Build history of the part. All positions in model axes, mm. A direction names the side the tool comes from. Round coordinates to 2 decimals unless told otherwise and drop trailing zeros. Write each loop counter-clockwise with the first axis right and the second up, starting at its lowest first coordinate (ties: lowest second). Pieces come first, ordered by that corner, then holes. Notation, with made-up numbers: (56, 35) - (103, 35) arc R15 ccw to (103, 55) - close; hole circle Ø3 at (86.25, 88). An arc over 180 degrees is marked (long way). One line per question, with ' | ' between items.
from build123d import *

# Parameters (mm, degrees)
BOSS_EXTRUDE1_DEPTH = 5
BOSS_EXTRUDE2_DEPTH = 1
SKETCH3_R           = 0.75
BOSS_EXTRUDE3_DEPTH = 2
CUT_EXTRUDE1_START  = -3
SKETCH4_R           = 0.75
CUT_EXTRUDE1_DEPTH  = 3


with BuildPart() as part:
    # Sketch1 → Boss-Extrude1 (new body)
    with BuildSketch(Plane.XY):
        Polygon((0, 57.735026919), (-50, 28.867513459), (-50, -28.867513459), (0, -57.735026919), (50, -28.867513459), (50, 28.867513459), align=None)
        Polygon((0, 54.270925304), (-47, 27.135462652), (-47, -27.135462652), (0, -54.270925304), (47, -27.135462652), (47, 27.135462652), align=None, mode=Mode.SUBTRACT)
    extrude(amount=BOSS_EXTRUDE1_DEPTH)

    # Sketch2 → Boss-Extrude2 (add)
    with BuildSketch(Plane(origin=(0, 0, 0), x_dir=(-1, 0, 0), z_dir=(0, 0, -1))):
        Polygon((-47, -27.135462652), (-47, 27.135462652), (0, 54.270925304), (47, 27.135462652), (47, -27.135462652), (0, -54.270925304), align=None)
    extrude(amount=-BOSS_EXTRUDE2_DEPTH)

    # Sketch3 → Boss-Extrude3 (add)
    # profile 1 of 6: a face of its own
    with BuildSketch(Plane.XY.offset(5)):
        with BuildLine():
            Line((1.5, 56.002976111), (1.5, 56.869001515))
            Line((1.5, 56.869001515), (0, 57.735026919))
            Line((0, 57.735026919), (-1.5, 56.869001515))
            Line((-1.5, 56.869001515), (-1.5, 56.002976111))
            ThreePointArc((-1.5, 56.002976111), (0, 54.502976111), (1.5, 56.002976111))
        make_face()
        with Locations((0, 56.002976111)):
            Circle(SKETCH3_R, mode=Mode.SUBTRACT)
    # profile 2 of 6: a face of its own
    with BuildSketch(Plane.XY.offset(5)):
        with BuildLine():
            Line((50, 27.135462652), (50, 28.867513459))
            Line((50, 28.867513459), (48.5, 29.733538863))
            Line((48.5, 29.733538863), (47.75, 29.300526161))
            ThreePointArc((47.75, 29.300526161), (47.200961894, 27.251488056), (49.25, 26.70244995))
            Line((49.25, 26.70244995), (50, 27.135462652))
        make_face()
        with Locations((48.5, 28.001488056)):
            Circle(SKETCH3_R, mode=Mode.SUBTRACT)
    # profile 3 of 6: a face of its own
    with BuildSketch(Plane.XY.offset(5)):
        with BuildLine():
            Line((50, -28.867513459), (50, -27.135462652))
            Line((50, -27.135462652), (49.25, -26.70244995))
            ThreePointArc((49.25, -26.70244995), (47.200961894, -27.251488056), (47.75, -29.300526161))
            Line((47.75, -29.300526161), (48.5, -29.733538863))
            Line((48.5, -29.733538863), (50, -28.867513459))
        make_face()
        with Locations((48.5, -28.001488056)):
            Circle(SKETCH3_R, mode=Mode.SUBTRACT)
    # profile 4 of 6: a face of its own
    with BuildSketch(Plane.XY.offset(5)):
        with BuildLine():
            Line((0, -57.735026919), (1.5, -56.869001515))
            Line((1.5, -56.869001515), (1.5, -56.002976111))
            ThreePointArc((1.5, -56.002976111), (0, -54.502976111), (-1.5, -56.002976111))
            Line((-1.5, -56.002976111), (-1.5, -56.869001515))
            Line((-1.5, -56.869001515), (0, -57.735026919))
        make_face()
        with Locations((0, -56.002976111)):
            Circle(SKETCH3_R, mode=Mode.SUBTRACT)
    # profile 5 of 6: a face of its own
    with BuildSketch(Plane.XY.offset(5)):
        with BuildLine():
            Line((-50, -28.867513459), (-48.5, -29.733538863))
            Line((-48.5, -29.733538863), (-47.75, -29.300526161))
            ThreePointArc((-47.75, -29.300526161), (-47.200961894, -27.251488056), (-49.25, -26.70244995))
            Line((-49.25, -26.70244995), (-50, -27.135462652))
            Line((-50, -27.135462652), (-50, -28.867513459))
        make_face()
        with Locations((-48.5, -28.001488056)):
            Circle(SKETCH3_R, mode=Mode.SUBTRACT)
    # profile 6 of 6: a face of its own
    with BuildSketch(Plane.XY.offset(5)):
        with BuildLine():
            Line((-47.75, 29.300526161), (-48.5, 29.733538863))
            Line((-48.5, 29.733538863), (-50, 28.867513459))
            Line((-50, 28.867513459), (-50, 27.135462652))
            Line((-50, 27.135462652), (-49.25, 26.70244995))
            ThreePointArc((-49.25, 26.70244995), (-47.200961894, 27.251488056), (-47.75, 29.300526161))
        make_face()
        with Locations((-48.5, 28.001488056)):
            Circle(SKETCH3_R, mode=Mode.SUBTRACT)
    extrude(amount=BOSS_EXTRUDE3_DEPTH)

    # Sketch4 → Cut-Extrude1 (cut)
    with BuildSketch(Plane.XY.offset(5).offset(CUT_EXTRUDE1_START)):
        with Locations((0, 56.002976111)):
            Circle(SKETCH4_R)
        with Locations((-48.5, 28.001488056)):
            Circle(SKETCH4_R)
        with Locations((-48.5, -28.001488056)):
            Circle(SKETCH4_R)
        with Locations((0, -56.002976111)):
            Circle(SKETCH4_R)
        with Locations((48.5, -28.001488056)):
            Circle(SKETCH4_R)
        with Locations((48.5, 28.001488056)):
            Circle(SKETCH4_R)
    extrude(amount=CUT_EXTRUDE1_DEPTH, mode=Mode.SUBTRACT)


solid = part.part
Q1. Saw through at A-A, the plane y = 23.5. List the corners of the cut face in (x, z), then the cut area to 3 significant figures.
Found:
outline: (-50, 0) - (50, 0) - (50, 5) - (47, 5) - (47, 1) - (-47, 1) - (-47, 5) - (-50, 5) - close | area: 124 mm^2
Q2. Drop flat-ended pins along their axis: pin 1 (2 mm diameter, centred on x = 13.5, y = -7, fed in from +Z); pin 2 (1.2 mm diameter, centred on x = 48.5, y = 28, fed in from +Z); pin 3 (1 mm diameter, centred on y = 56.5, z = 6.5, fed in from -X). Give the stop position or say it passes through.
Found:
pin 1: z = 1 | pin 2: z = 2 | pin 3: x = -1.5
Q3. Pull direction X, two halves, no side cores. Call faces 1 (the flat face through (50, 0, 2)), 2 (the flat face through (-47, 0, 3)), 3 (the flat face through (48, -29, 7)), 4 (the flat face through (23.829, 40.513, 2.972)): +X half, -X half, draft (parallel to the pull), parting line (faces both ways), or undercut.
Found:
face 1: +X half | face 2: undercut | face 3: draft | face 4: undercut
Q4. Saw through at B-B, the plane x = 21. List the corners of the cut face in (y, z), then the cut area to 3 significant figures.
Found:
outline: (-45.61, 0) - (45.61, 0) - (45.61, 5) - (42.15, 5) - (42.15, 1) - (-42.15, 1) - (-42.15, 5) - (-45.61, 5) - close | area: 119 mm^2
Q5. Drill centre lines: L1, parallel to Y at x = -48.5, z = 5.35; L2, parallel to Y at x = 0, z = 3.5; L3, parallel to X at y = -2, z = 4.75. Where is each one in solid material? Low to high. Write a range as from..to.
Found:
L1: -29.73..-28.75, -27.25..-26.5, 26.5..27.25, 28.75..29.73 | L2: -57.74..-56.75, -55.25..-54.27, 54.27..55.25, 56.75..57.74 | L3: -50..-47, 47..50
Q6. Which spindle directions (+Z, -Z, +X, -X, +Y, -Y) get a long thin tool onto all of the face, cutting with end or side? Do faces 5 (the flat face through (-23.829, -40.513, 2.972)), 6 (the flat face through (-50, 0, 2)). Say none if no direction does.
Found:
face 5: +Z | face 6: +Z, -Z, -X, +Y, -Y
